Geometry: final body of the model. Coordinates: model frame, mm. A direction names the side the tool comes from. Round coordinates to 2 decimals unless told otherwise and drop trailing zeros. Write each loop counter-clockwise with the first axis right and the second up, starting at its lowest first coordinate (ties: lowest second). Pieces come first, ordered by that corner, then holes. Notation, with made-up numbers: M 78.25,25 L 119.25,25 A31 cw 119.25,50 Z; hole C -19.5,-14 d8. An arc over 180 degrees is marked long. Answer as CSV lines item,"result". Start each with the question number.
Q1. Section query D-D on y = -134. Output: boundary loops of the cut face in (x, z), and give its area (3 significant figures).
Q2. Section query C-C on x = -113.5. Output: boundary loops of the cut face in (y, z).
Q3. Section query A-A on y = 159. Output: boundary loops of the cut face in (x, z).
Q4. Mould query, pull axis X, two halves, no side actions, for faces 3 (the flat face through (-3, 40, 0)), 4 (the cylindrical face through (-7.47, -199.86, 2.46)), 5 (the flat face through (39.8, 51.56, 2.54)). Classes: pulls with the +X half, pulls with the -X half, needs draft (parallel to the pull), parting line crosses it, or undercut.
Q5. Ray query, probe 1 along Y at (x, z) = (20, 3.75); probe 2 along X at (y, z) = (72, 2.9); probe 3 along Y at (x, z) = (160.5, 3.6). Return the intervals inside material, ascending.
Q6. First-contact query: pin 1 (2.5 mm diameter, centred on x = -27.66, y = -37.39, fed in from +Z); pin 2 (1.5 mm diameter, centred on x = -58.5, z = 0.5, fed in from -Y); pin 3 (2 mm diameter, centred on x = 20, z = 1.5, fed in from +Y). Flat tips, straight axial feed; report the tip coordinate or a pass-through.
Q7. Reachability of faces 1 (the flat face through (-159.936, 92.982, 2.465)), 2 (the flat face through (-3, 40, 5)) from +Z, -Z, +X, -X, +Y, -Y: full face, straight path, thin tool, end or side. Return the list, or none.
Q8. Section query B-B on x = 0. Output: boundary loops of the cut face in (y, z), and give its area (3 significant figures).
```python
from build123d import *

# Parameters (mm, degrees)
BOSS_EXTRUDE1_DEPTH = 5
SKETCH2_R           = 6
CUT_EXTRUDE1_DEPTH  = 6
CUT_EXTRUDE3_DEPTH  = 6
SKETCH4_R           = 1.5
CUT_EXTRUDE4_DEPTH  = 6
SKETCH5_R           = 2
CUT_EXTRUDE5_DEPTH  = 6
SKETCH6_R           = 2.1
CUT_EXTRUDE6_DEPTH  = 6


with BuildPart() as part:
    # Sketch1 → Boss-Extrude1 (new body)
    with BuildSketch(Plane.XY):
        with BuildLine():
            ThreePointArc((-133.768727702, -148.680622439), (-5.497740296, -199.924422849), (125.395583095, -155.807405923))
            ThreePointArc((125.395583095, -155.807405923), (105.414180622, -62.702389546), (196.766071989, -35.820565518))
            ThreePointArc((196.766071989, -35.820565518), (173.617953569, 99.281449418), (68.919790336, 187.75))
            ThreePointArc((68.919790336, 187.75), (0, 130), (-68.919790336, 187.75))
            ThreePointArc((-68.919790336, 187.75), (-171.192781262, 103.407116021), (-198.254420354, -26.366357541))
            ThreePointArc((-198.254420354, -26.366357541), (-113.788656518, -59.99087954), (-133.768727702, -148.680622439))
        make_face()
    extrude(amount=BOSS_EXTRUDE1_DEPTH)

    # Sketch2 → Cut-Extrude1 (cut, through all)
    with BuildSketch(Plane.XY.offset(5)):
        Circle(SKETCH2_R)
    extrude(amount=-CUT_EXTRUDE1_DEPTH, mode=Mode.SUBTRACT)

    # Sketch3 → Cut-Extrude3 (cut, through all)
    with BuildSketch(Plane.XY.offset(5)):
        Polygon((-131.763323944, 111.527693705), (-66.967361155, 73.758881092), (-74.521123677, 60.799688534), (-22.684353446, 30.584638444), (-37.791878491, 4.666253328), (-89.628648723, 34.881303419), (-97.182411245, 21.922110861), (-161.978374035, 59.690923474), align=None)
        Polygon((162.467477946, 58.34653897), (97.360745358, 21.115995438), (89.914636652, 34.137341956), (37.829250581, 4.352907131), (22.937033168, 30.395600166), (75.022419239, 60.180034991), (67.576310532, 73.201381509), (132.683043121, 110.431925041), align=None)
        Polygon((-30.704154002, -169.874232675), (-30.393384203, -94.874876531), (-15.393512974, -94.93703049), (-15.144897135, -34.937545574), (14.854845323, -35.061853494), (14.606229484, -95.06133841), (29.606100713, -95.12349237), (29.295330914, -170.122848514), align=None)
    extrude(amount=-CUT_EXTRUDE3_DEPTH, mode=Mode.SUBTRACT)

    # Sketch4 → Cut-Extrude4 (cut, through all)
    with BuildSketch(Plane.XY.offset(5)):
        with Locations((-57.426994444, 65.304213564)):
            Circle(SKETCH4_R)
        with Locations((-18.54941677, 42.642925996)):
            Circle(SKETCH4_R)
        with Locations((-46.246546019, -4.874113383)):
            Circle(SKETCH4_R)
        with Locations((-85.124123693, 17.787174185)):
            Circle(SKETCH4_R)
        with Locations((85.268605142, 17.081129269)):
            Circle(SKETCH4_R)
        with Locations((46.204565589, -5.25719685)):
            Circle(SKETCH4_R)
        with Locations((18.902166999, 42.487740382)):
            Circle(SKETCH4_R)
        with Locations((57.966206552, 64.826066501)):
            Circle(SKETCH4_R)
        with Locations((-27.841610699, -82.385342833)):
            Circle(SKETCH4_R)
        with Locations((-27.655148819, -37.385729146)):
            Circle(SKETCH4_R)
        with Locations((27.34437902, -37.613626999)):
            Circle(SKETCH4_R)
        with Locations((27.157917141, -82.613240686)):
            Circle(SKETCH4_R)
        Polygon((-75.583756982, 9.332506656), (-73.065836141, 13.652237509), (-55.786912731, 3.580554145), (-58.304833571, -0.739176707), align=None)
        Polygon((-47.886627732, 56.849546035), (-45.368706892, 61.169276888), (-28.089783481, 51.097593524), (-30.607704322, 46.777862672), align=None)
        Polygon((45.874066336, 60.791200332), (48.356102572, 56.450751492), (30.994307215, 46.522606551), (28.512270979, 50.86305539), align=None)
        Polygon((73.176464926, 13.0462631), (75.658501162, 8.705814261), (58.296705805, -1.222330681), (55.814669569, 3.118118158), align=None)
        Polygon((29.709690646, -70.123706988), (24.709733569, -70.102989001), (24.792605516, -50.103160696), (29.792562592, -50.123878683), align=None)
        Polygon((-25.289837194, -69.895809136), (-30.28979427, -69.875091149), (-30.206922324, -49.875262844), (-25.206965248, -49.89598083), align=None)
    extrude(amount=-CUT_EXTRUDE4_DEPTH, mode=Mode.SUBTRACT)

    # Sketch5 → Cut-Extrude5 (cut, through all)
    with BuildSketch(Plane.XY.offset(5)):
        with Locations((71.464466094, 128.964466094)):
            Circle(SKETCH5_R)
        with Locations((71.464466094, 86.035533906)):
            Circle(SKETCH5_R)
        with Locations((28.535533906, 86.035533906)):
            Circle(SKETCH5_R)
        with Locations((28.535533906, 128.964466094)):
            Circle(SKETCH5_R)
    extrude(amount=-CUT_EXTRUDE5_DEPTH, mode=Mode.SUBTRACT)

    # Sketch6 → Cut-Extrude6 (cut, through all)
    with BuildSketch(Plane(origin=(0, 0, 0), x_dir=(-1, 0, 0), z_dir=(0, 0, -1))):
        with Locations((141.303690655, 119.982361234)):
            Circle(SKETCH6_R)
        with Locations((174.036661587, 63.825860149)):
            Circle(SKETCH6_R)
        with Locations((33.255927507, -182.363766373)):
            Circle(SKETCH6_R)
        with Locations((-31.743514485, -182.633100198)):
            Circle(SKETCH6_R)
        with Locations((-174.559618162, 62.381405139)):
            Circle(SKETCH6_R)
        with Locations((-142.293147101, 118.807240049)):
            Circle(SKETCH6_R)
        Polygon((-148.810049506, 102.374650994), (-153.150498345, 104.85668723), (-168.042715757, 78.813994194), (-163.702266918, 76.331957959), align=None)
        Polygon((163.064073217, 77.685957713), (167.38380407, 80.203878554), (152.276279025, 106.12226367), (147.956548172, 103.604342829), align=None)
        Polygon((-14.254023712, -180.060608707), (-14.233305725, -185.060565784), (15.766436733, -184.936257864), (15.745718746, -179.936300788), align=None)
    extrude(amount=-CUT_EXTRUDE6_DEPTH, mode=Mode.SUBTRACT)


solid = part.part
```
Entries:
1,outline,"M -119.24,0 L -30.56,0 L -30.56,5 L -119.24,5 Z; M 29.45,0 L 105.25,0 L 105.25,5 L 29.45,5 Z"
1,area,"822 mm^2"
2,outline,"M -164.67,0 L -124.73,0 L -124.73,5 L -164.67,5 Z; M -60.54,0 L 31.43,0 L 31.43,5 L -60.54,5 Z; M 100.88,0 L 164.67,0 L 164.67,5 L 100.88,5 Z"
3,outline,"M -121.32,0 L -56.74,0 L -56.74,5 L -121.32,5 Z; M 56.74,0 L 121.32,0 L 121.32,5 L 56.74,5 Z"
4,face 3,"needs draft"
4,face 4,"parting line crosses it"
4,face 5,"undercut"
5,probe 1,"y = -199 to -170.08, -95.08 to 41.47, 43.51 to 132.92"
5,probe 2,"x = -186.59 to -154.8, -67.99 to 68.26, 154.66 to 186.59"
5,probe 3,"y = -28.67 to 57.22, 61.79 to 81.93, 92 to 119.33"
6,pin 1,"passes through"
6,pin 2,"stops at y = -191.48"
6,pin 3,"stops at y = 133.22"
7,face 1,"+Z, -Z"
7,face 2,"+Z, +X, -X, +Y, -Y"
8,outline,"M -200,0 L -185,0 L -185,5 L -200,5 Z; M -180,0 L -170,0 L -170,5 L -180,5 Z; M -35,0 L -6,0 L -6,5 L -35,5 Z; M 6,0 L 130,0 L 130,5 L 6,5 Z"
8,area,"890 mm^2"
